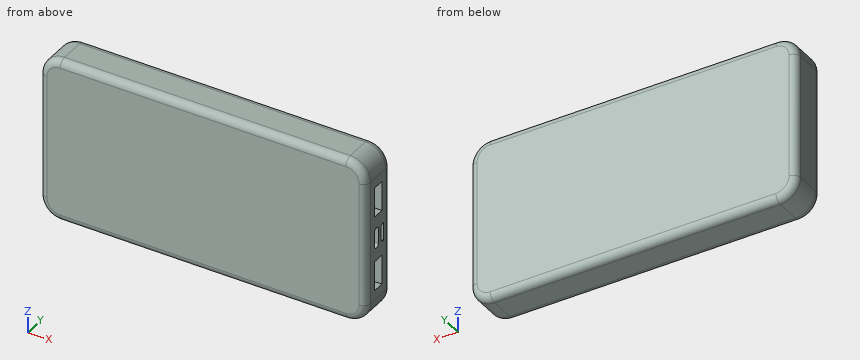
```python
from build123d import *

# Parameters (mm, degrees)
SKETCH1_W           = 136.5
SKETCH1_H           = 69
BOSS_EXTRUDE1_DEPTH = 16.25
FILLET1_R           = 8.5
FILLET2_R           = 3
SKETCH2_W           = 12.4
SKETCH2_H           = 5
CUT_EXTRUDE1_DEPTH  = 12
CUT_EXTRUDE2_DEPTH  = 5
CUT_EXTRUDE3_DEPTH  = 4


with BuildPart() as part:
    # Sketch1 → Boss-Extrude1 (new body)
    with BuildSketch(Plane(origin=(0, 0, 0), x_dir=(1, 0, 0), z_dir=(0, 1, 0))):
        with Locations((68.25, -34.5)):
            Rectangle(SKETCH1_W, SKETCH1_H)
    extrude(amount=BOSS_EXTRUDE1_DEPTH)

    # Fillet1
    fillet1_edges = [part.edges().sort_by_distance(p)[0] for p in [
        (0, 8.125, 0),
        (136.5, 8.125, 0),
        (136.5, 8.125, 69),
        (0, 8.125, 69),
    ]]
    fillet(fillet1_edges, radius=FILLET1_R)

    # Fillet2
    fillet2_edges = [part.edges().sort_by_distance(p)[0] for p in [
        (0, 0, 34.5),
        (0, 16.25, 34.5),
        (68.25, 0, 0),
        (136.5, 0, 34.5),
        (68.25, 0, 69),
        (134.01040764, 0, 66.51040764),
        (134.01040764, 0, 2.48959236),
        (2.48959236, 0, 66.51040764),
        (2.48959236, 0, 2.48959236),
        (68.25, 16.25, 0),
        (68.25, 16.25, 69),
        (136.5, 16.25, 34.5),
        (134.01040764, 16.25, 66.51040764),
        (134.01040764, 16.25, 2.48959236),
        (2.48959236, 16.25, 66.51040764),
        (2.48959236, 16.25, 2.48959236),
    ]]
    fillet(fillet2_edges, radius=FILLET2_R)

    # Sketch2 → Cut-Extrude1 (cut)
    with BuildSketch(Plane(origin=(136.5, 0, 0), x_dir=(0, 0, -1), z_dir=(1, 0, 0))):
        with Locations((-18.7, 8.125)):
            Rectangle(SKETCH2_W, SKETCH2_H)
        with Locations((-50.3, 8.125)):
            Rectangle(SKETCH2_W, SKETCH2_H)
    extrude(amount=-CUT_EXTRUDE1_DEPTH, mode=Mode.SUBTRACT)

    # Sketch3 → Cut-Extrude2 (cut)
    with BuildSketch(Plane(origin=(136.5, 0, 0), x_dir=(0, 0, -1), z_dir=(1, 0, 0))):
        with BuildLine():
            Line((-37.575, 5.625), (-31.425, 5.625))
            ThreePointArc((-31.425, 5.625), (-30.125, 6.925), (-31.425, 8.225))
            Line((-31.425, 8.225), (-37.575, 8.225))
            ThreePointArc((-37.575, 8.225), (-38.875, 6.925), (-37.575, 5.625))
        make_face()
    extrude(amount=-CUT_EXTRUDE2_DEPTH, mode=Mode.SUBTRACT)

    # Sketch4 → Cut-Extrude3 (cut)
    with BuildSketch(Plane(origin=(136.5, 0, 0), x_dir=(0, 0, -1), z_dir=(1, 0, 0))):
        with BuildLine():
            Line((-37.344933438, 10), (-31.655066562, 10))
            ThreePointArc((-31.655066562, 10), (-31.224884235, 10.135635967), (-30.950297096, 10.493484893))
            Line((-30.950297096, 10.493484893), (-30.615076845, 11.414494964))
            ThreePointArc((-30.615076845, 11.414494964), (-30.645211989, 11.643394109), (-30.85, 11.75))
            Line((-30.85, 11.75), (-38.15, 11.75))
            ThreePointArc((-38.15, 11.75), (-38.354788011, 11.643394109), (-38.384923155, 11.414494964))
            Line((-38.384923155, 11.414494964), (-38.049702904, 10.493484893))
            ThreePointArc((-38.049702904, 10.493484893), (-37.775115765, 10.135635967), (-37.344933438, 10))
        make_face()
    extrude(amount=-CUT_EXTRUDE3_DEPTH, mode=Mode.SUBTRACT)


solid = part.part
```
Model file for the job. Use its own axes, mm. Give positions to 0.01 mm unless a question says otherwise; leave off trailing zeros. Write each loop counter-clockwise with the first axis right and the second up, starting at its lowest first coordinate (ties: lowest second). Pieces come first, ordered by that corner, then holes. Notation, with made-up numbers: (32, -6) - (55, -6) arc R18 cw to (55, 29) - close; hole circle Ø11 at (-11.75, 12.25). An arc over 180 degrees is marked (long way). One line per question, with ' | ' between items. Start each with the question number.
(1) Slice it at A-A on z = 14. Write the cut outline in (x, y) (3 decimals), plus the area to 3 significant figures.
(2) Slice it at B-B on y = 1.5. Write the cut outline in (x, z).
(3) Wall check: line 1 along X through (y, z) = (13.5, 45.5); line 2 along X through (y, z) = (9, 53); line 3 along Z through (x, y) = (13.5, 2). Give the ranges that are in metal, low to high. Write a range as from..to.
(4) Pin check, flat tips, straight feed: P1, Ø2.5, axis at y = 9, z = 19.5, coming from the +X side; P2, Ø1.9, axis at y = 10.5, z = 33.5, coming from the +X side; P3, Ø1.3, axis at y = 7.5, z = 33.5, coming from the +X side; P4, Ø2.5, axis at x = 135, z = 35.5, coming from the +Y side. Stop position of each tip, or through.
Results below:
1) outline: (0, 3) arc R3 ccw to (3, 0) - (133.5, 0) arc R3 ccw to (136.5, 3) - (136.5, 5.625) - (124.5, 5.625) - (124.5, 10.625) - (136.5, 10.625) - (136.5, 13.25) arc R3 ccw to (133.5, 16.25) - (3, 16.25) arc R3 ccw to (0, 13.25) - close | area: 2,150 mm^2
2) outline: (0.4, 8.5) arc R8.1 ccw to (8.5, 0.4) - (128, 0.4) arc R8.1 ccw to (136.1, 8.5) - (136.1, 60.5) arc R8.1 ccw to (128, 68.6) - (8.5, 68.6) arc R8.1 ccw to (0.4, 60.5) - close
3) line 1: 0.01..136.49 | line 2: 0..124.5 | line 3: 0.17..68.83
4) P1: x = 124.5 | P2: x = 136.5 | P3: x = 131.5 | P4: y = 16.24
